For this review, take the finished solid that the model builds, in its own axes (mm). A direction names the side the tool comes from. Coordinates: 2 decimals unless noted, no trailing zeros. Order: outer loops, then holes, each group sorted by start corner. A loop starts at its lowest first (then second) coordinate and runs counter-clockwise, first axis right, second up.
from build123d import *

# Parameters (mm, degrees)
SKETCH1_W               = 550
SKETCH1_H               = 200
EXTRUDE1_DEPTH          = 15
SKETCH3_W               = 15
SKETCH3_H               = 200
EXTRUDE2_DEPTH          = 50
CUT_EXTRUDE3_DEPTH      = 536
CUT_EXTRUDE3_DEPTH_BACK = 16
CUT_EXTRUDE4_DEPTH      = 536
CUT_EXTRUDE4_DEPTH_BACK = 16
SKETCH8_R               = 6.5
CUT_EXTRUDE5_DEPTH      = 16


with BuildPart() as part:
    # Sketch1 → Extrude1 (new body)
    with BuildSketch(Plane(origin=(0, 0, 0), x_dir=(1, 0, 0), z_dir=(0, 1, 0))):
        with Locations((275, 0)):
            Rectangle(SKETCH1_W, SKETCH1_H)
    extrude(amount=-EXTRUDE1_DEPTH)

    # Sketch3 → Extrude2 (add)
    with BuildSketch(Plane(origin=(0, 0, 0), x_dir=(-1, 0, 0), z_dir=(0, 1, 0))):
        with Locations((-542.5, 0)):
            Rectangle(SKETCH3_W, SKETCH3_H)
    extrude(amount=EXTRUDE2_DEPTH)

    # Sketch4 → Cut-Extrude3 (cut, two sides)
    with BuildSketch(Plane.ZY.offset(-535)) as cut_extrude3_sk:
        Polygon((-100, 50), (-100, 0), (-25, 50), align=None)
    extrude(amount=CUT_EXTRUDE3_DEPTH, mode=Mode.SUBTRACT)
    extrude(cut_extrude3_sk.sketch, amount=-CUT_EXTRUDE3_DEPTH_BACK, mode=Mode.SUBTRACT)

    # Sketch7 → Cut-Extrude4 (cut, two sides)
    with BuildSketch(Plane.ZY.offset(-535)) as cut_extrude4_sk:
        Polygon((451.383627881, -234.255751921), (100, 0), (25, 50), (-326.383627881, 284.255751921), (142.12787596, 987.023007684), (919.895131723, 468.511503842), align=None)
    extrude(amount=CUT_EXTRUDE4_DEPTH, mode=Mode.SUBTRACT)
    extrude(cut_extrude4_sk.sketch, amount=-CUT_EXTRUDE4_DEPTH_BACK, mode=Mode.SUBTRACT)

    # Sketch8 → Cut-Extrude5 (cut, through all)
    with BuildSketch(Plane(origin=(0, 0, 0), x_dir=(-1, 0, 0), z_dir=(0, 1, 0))):
        with Locations((-50, -60)):
            Circle(SKETCH8_R)
        with Locations((-200, -60)):
            Circle(SKETCH8_R)
        with Locations((-50, 60)):
            Circle(SKETCH8_R)
        with Locations((-200, 60)):
            Circle(SKETCH8_R)
    extrude(amount=-CUT_EXTRUDE5_DEPTH, mode=Mode.SUBTRACT)


solid = part.part
1. Clearance check with flat-ended pins moving along their axes: pin 1 Ø21 at (x, z) = (50, 60) entering from -Y; pin 2 Ø2 at (x, z) = (71.5, -72.5) entering from +Y. State where each tip first meets the part, or that it passes through.
Answer below:
pin 1: stops at y = -15
pin 2: stops at y = 0
2. Take a section at C-C, the plane y = 45. Give the boundary of the cut face in (x, z).
Answer below:
outline: (535, -32.5) - (550, -32.5) - (550, 32.5) - (535, 32.5) - close
3. The part is to be moulded in two halves that separate along Z. For faces 3 (the face through (205.158, -7.395, -63.955)), 4 (the face through (542.395, 24.65, -63.025)), 5 (the face through (271, -15, -1)), say which applies: +Z half, -Z half, draft (parallel to the pull), parting line (faces both ways), or undercut.
Answer below:
face 3: undercut
face 4: -Z half
face 5: draft
4. Take a section at A-A, the plane x = 50. Give the boundary of the cut face in (y, z).
Answer below:
outline: (-15, -100) - (0, -100) - (0, -66.5) - (-15, -66.5) - close; (-15, -53.5) - (0, -53.5) - (0, 53.5) - (-15, 53.5) - close; (-15, 66.5) - (0, 66.5) - (0, 100) - (-15, 100) - close
5. Machinability: for faces 1 (the face through (264, 0, -1)), 2 (the face through (51.409, -7.395, 53.655)), which of the approach directions +Z, -Z, +X, -X, +Y, -Y give a long, thin tool a straight path to every point of the face, cutting with its end or side? Answer none if there is none.
Answer below:
face 1: +Z, -Z, -X, +Y
face 2: +Y, -Y
6. Take a section at B-B, the plane z = 60. Give the boundary of the cut face in (x, y).
Answer below:
outline: (0, -15) - (43.5, -15) - (43.5, 0) - (0, 0) - close; (56.5, -15) - (193.5, -15) - (193.5, 0) - (56.5, 0) - close; (206.5, -15) - (550, -15) - (550, 26.67) - (535, 26.67) - (535, 0) - (206.5, 0) - close
7. Take a section at D-D, the plane z = 82. Give the boundary of the cut face in (x, y), plus the area to 3 significant figures.
Answer below:
outline: (0, -15) - (550, -15) - (550, 12) - (535, 12) - (535, 0) - (0, 0) - close
area: 8,430 mm2
8. To check wall thickness, follow L1, parallel to Z at x = 200, y = -7; L2, parallel to Y at x = 119.5, z = -31; L3, parallel to X at y = 1, z = -2.5. State the ranges of each line that lie inside material, in increasing order.
Answer below:
L1: z = -100 to -66.5, -53.5 to 53.5, 66.5 to 100
L2: y = -15 to 0
L3: x = 535 to 550
